Read the model definition and answer for the solid it produces. Units are mm, in the model's axes. A direction names the side the tool comes from. Give positions to 0.01 mm unless a question says otherwise; leave off trailing zeros. Write each loop counter-clockwise with the first axis right and the second up, starting at its lowest first coordinate (ties: lowest second). Pieces come first, ordered by that corner, then holes. Notation, with made-up numbers: M 17.25,-19 L 51.25,-19 A18 ccw 51.25,-3 Z; hole C -27,70.25 d4. An arc over 180 degrees is marked long. Answer as CSV lines item,"result". Start each with the question number.
```python
from build123d import *

# Parameters (mm, degrees)
BOSS_EXTRUDE1_DEPTH = 19.5
SKETCH2_W           = 8
SKETCH2_H           = 4
BOSS_EXTRUDE2_DEPTH = 7
SKETCH3_R           = 4.5
BOSS_EXTRUDE3_DEPTH = 5.3
SKETCH4_W           = 9
SKETCH4_H           = 9
BOSS_EXTRUDE4_DEPTH = 1
BOSS_EXTRUDE5_DEPTH = 2


with BuildPart() as part:
    # Sketch1 → Boss-Extrude1 (new body)
    with BuildSketch(Plane(origin=(0, 0, 0), x_dir=(0, 0, -1), z_dir=(1, 0, 0))):
        Polygon((0, 0), (45, 0), (45, 25), (52, 25), (52, 30.8), (45, 30.8), (45, 36.3), (0, 36.3), (0, 30.8), (-7, 30.8), (-7, 25), (0, 25), align=None)
    extrude(amount=BOSS_EXTRUDE1_DEPTH)

    # Sketch2 → Boss-Extrude2 (add)
    with BuildSketch(Plane.XY):
        with Locations((9.75, 2)):
            Rectangle(SKETCH2_W, SKETCH2_H)
    extrude(amount=BOSS_EXTRUDE2_DEPTH)

    # Sketch3 → Boss-Extrude3 (add)
    with BuildSketch(Plane(origin=(0, 36.3, 0), x_dir=(1, 0, 0), z_dir=(0, 1, 0))):
        with Locations(Location((9.75, 10, 0), (0, 0, 90))):
            Circle(SKETCH3_R)
    extrude(amount=BOSS_EXTRUDE3_DEPTH)

    # Sketch4 → Boss-Extrude4 (add)
    with BuildSketch(Plane(origin=(0, 41.6, 0), x_dir=(1, 0, 0), z_dir=(0, 1, 0))):
        with Locations((9.75, 10)):
            Rectangle(SKETCH4_W, SKETCH4_H)
    extrude(amount=BOSS_EXTRUDE4_DEPTH)

    # Sketch5 → Boss-Extrude5 (add)
    with BuildSketch(Plane(origin=(0, 42.6, 0), x_dir=(1, 0, 0), z_dir=(0, 1, 0))):
        Polygon((5.25, 14.5), (14.25, 14.5), (34.95, 12.5), (34.95, 10), (34.95, 7.5), (14.25, 5.5), (5.25, 5.5), align=None)
    extrude(amount=BOSS_EXTRUDE5_DEPTH)


solid = part.part
```
1. Find section B-B on x = 15.5. Determine the outline of the cut face in (y, z), then the cut area to 3 significant figures.
2. Find section D-D on z = -48. Determine the outline of the cut face in (x, y).
3. Find section A-A on z = 1. Determine the outline of the cut face in (x, y), then the cut area to 3 significant figures.
4. Determine the mould class of faces 1 (the face through (6, 41.6, -13)), 2 (the face through (13.75, 2, 3)), 3 (the face through (10, 30.8, -49)), 4 (the face through (10, 4, 3)) for opening direction Y: +Y half, -Y half, draft (parallel to the pull), parting line (faces both ways), or undercut.
5. Find section C-C on y = 40.5. Determine the outline of the cut face in (x, z).
6. For faces 5 (the face through (10, 43, -5.5)), 6 (the face through (5.25, 43, -10)), 7 (the face through (24.455, 43.586, -13.514)), determine the directions among +Z, -Z, +X, -X, +Y, -Y from which every point of the face is accessible in a straight line to the end or side of a thin tool.
7. Given pin 1 (1.3 mm diameter, centred on x = 8.5, z = -13, fed in from -Y); pin 2 (1 mm diameter, centred on x = 8.5, z = -37.5, fed in from +Y); pin 3 (5 mm diameter, centred on y = 36.5, z = -32, fed in from +X); pin 4 (4.5 mm diameter, centred on y = 2, z = 3.5, fed in from +X), each flat-ended and moving along its own axis, determine where each tip first touches the part or whether it passes through.
8. Find the intervals of material crossed by line 1 (X direction, y = 19, z = -17); line 2 (Z direction, x = 9, y = 17); line 3 (Y direction, x = 17, z = -43.5), in increasing order. Write a range as [from, to].
Computed:
1,outline,"M 0,-45 L 25,-45 L 25,-52 L 30.8,-52 L 30.8,-45 L 36.3,-45 L 36.3,0 L 30.8,0 L 30.8,7 L 25,7 L 25,0 L 0,0 Z; M 42.6,-14.38 L 44.6,-14.38 L 44.6,-5.62 L 42.6,-5.62 Z"
1,area,"1,730 mm^2"
2,outline,"M 0,25 L 19.5,25 L 19.5,30.8 L 0,30.8 Z"
3,outline,"M 0,25 L 19.5,25 L 19.5,30.8 L 0,30.8 Z; M 5.75,0 L 13.75,0 L 13.75,4 L 5.75,4 Z"
3,area,"145 mm^2"
4,face 1,"undercut"
4,face 2,"draft"
4,face 3,"+Y half"
4,face 4,"undercut"
5,outline,"C 9.75,-10 d9"
6,face 5,"+Z, +X, -X, +Y"
6,face 6,"+Z, -Z, -X, +Y"
6,face 7,"-Z, +X, +Y"
7,pin 1,"stops at y = 0"
7,pin 2,"stops at y = 36.3"
7,pin 3,"stops at x = 19.5"
7,pin 4,"stops at x = 13.75"
8,line 1,"x = [0, 19.5]"
8,line 2,"z = [-45, 0]"
8,line 3,"y = [0, 36.3]"
